Drawing for the job (mm, zero at the part's lowest x, y, z). A direction names the side the tool comes from. Give positions to 0.01 mm unless a question says otherwise; leave off trailing zeros. Order: outer loops, then holes, each group sorted by start corner. A loop starts at its lowest first (then second) coordinate and runs counter-clockwise, first axis right, second up. Notation, with made-up numbers: (36.5, 13) -> (53.5, 13) arc R27 cw to (53.5, 47) -> close; hole circle Ø10 at (15, 48). An arc over 180 degrees is marked (long way). One line per item, written item: value. Start each with the question number.
(1) Pin check, flat tips, straight feed: pin 1 (5 mm diameter, centred on x = 8.5, y = 14, fed in from -Z); pin 2 (3 mm diameter, centred on x = 4.5, y = 6, fed in from +Z); pin 3 (2 mm diameter, centred on x = 2.5, y = 9, fed in from -Z); pin 4 (4 mm diameter, centred on y = 11.11, z = 11.11, fed in from -X). Stop position of each tip, or through.
(2) Two-plate mould, pull along Y, no slides. Class the marked faces 3, 4 and 5: +Y half, -Y half, draft (parallel to the pull), parting line (faces both ways), or undercut.
(3) Saw through at C-C on z = 6.5. Give the cut face in (x, y) (1 decimal).
(4) Saw through at A-A on y = 11. Give the cut face in (x, z) (1 decimal).
(5) Probe line 1 (Y direction, x = 4.75, z = 11.25) (1 decimal); line 2 (X direction, y = 17.5, z = 4); line 3 (Y direction, x = 1, z = 11.75). List the from-to ranges inside material, lowest first.
(6) Saw through at B-B on z = 10. Give the cut face in (x, y) (1 decimal), plus the area to 3 significant figures.
(7) Which spindle directions (+Z, -Z, +X, -X, +Y, -Y) get a long thin tool onto all of the face, cutting with end or side? Do the marked faces 1 and 2. Say none if no direction does.
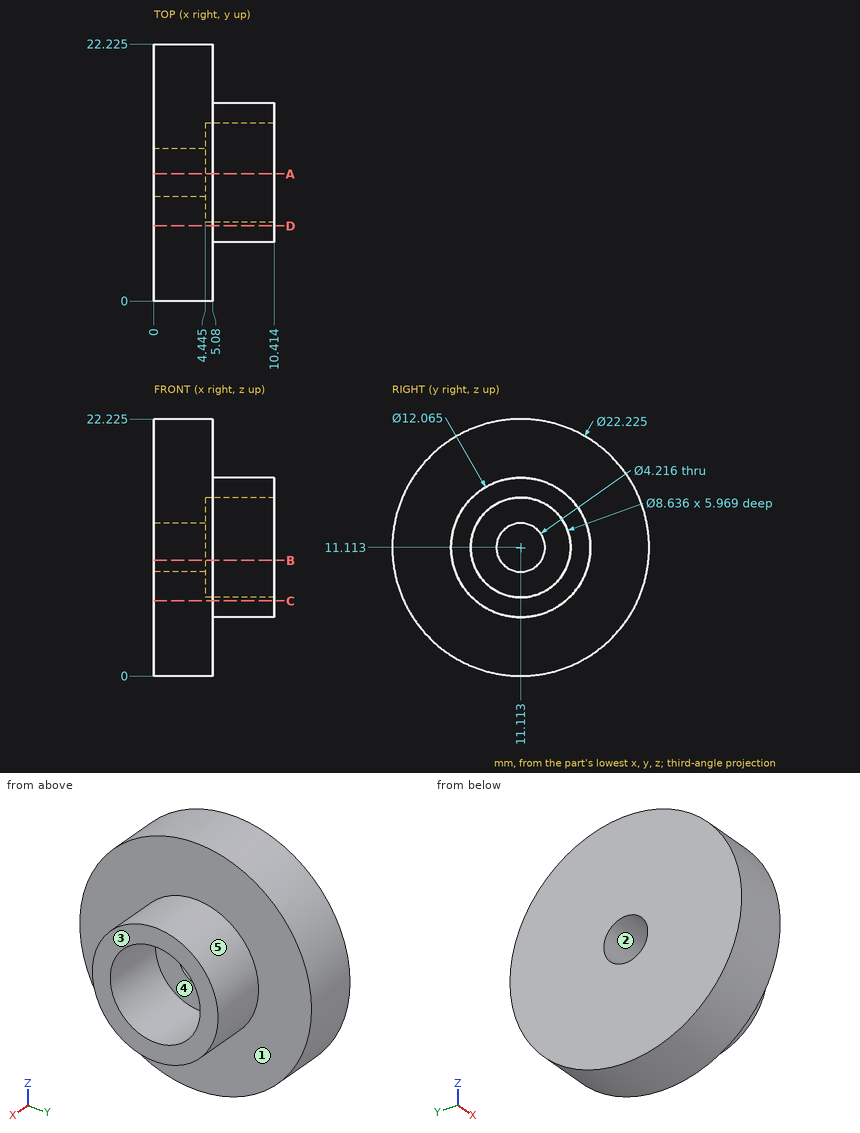
Results below:
1. pin 1: stops at z = 5.09
1. pin 2: stops at z = 21.62
1. pin 3: stops at z = 0.06
1. pin 4: passes through
2. face 3: draft
2. face 4: undercut
2. face 5: parting line
3. outline: (0, 1) -> (5.1, 1) -> (5.1, 7.2) -> (10.4, 7.2) -> (10.4, 15) -> (5.1, 15) -> (5.1, 21.2) -> (0, 21.2) -> close
4. outline: (0, 0) -> (5.1, 0) -> (5.1, 5.1) -> (10.4, 5.1) -> (10.4, 6.8) -> (4.4, 6.8) -> (4.4, 9) -> (0, 9) -> close; (0, 13.2) -> (4.4, 13.2) -> (4.4, 15.4) -> (10.4, 15.4) -> (10.4, 17.1) -> (5.1, 17.1) -> (5.1, 22.2) -> (0, 22.2) -> close
5. line 1: y = 0 to 6.8, 15.4 to 22.2
5. line 2: x = 0 to 5.08
5. line 3: y = 0.02 to 9.1, 13.12 to 22.21
6. outline: (0, 0.1) -> (5.1, 0.1) -> (5.1, 5.2) -> (10.4, 5.2) -> (10.4, 6.9) -> (4.4, 6.9) -> (4.4, 9.3) -> (0, 9.3) -> close; (0, 12.9) -> (4.4, 12.9) -> (4.4, 15.3) -> (10.4, 15.3) -> (10.4, 17) -> (5.1, 17) -> (5.1, 22.2) -> (0, 22.2) -> close
6. area: 110 mm²
7. face 1: +X
7. face 2: +X, -X
